```python
from build123d import *
from OCP.BRepFilletAPI import BRepFilletAPI_MakeChamfer

# Parameters (mm, degrees)
SKETCH9_R                    = 2
BOSS_EXTRUDE3_DEPTH          = 16
SKETCH10_R                   = 2
CUT_EXTRUDE7_DEPTH           = 14
SKETCH11_W                   = 7
SKETCH11_H                   = 26.686138344
CUT_EXTRUDE8_DEPTH           = 28
FILLET1_R                    = 2
CHAMFER1_SIZE                = 2.5
CHAMFER1_SIZE2               = 4.365846821
CHAMFER1_SIZE2_2             = 4.330127019
EXTRUDE1_DEPTH               = 3
EXTRUDE1_DEPTH_BACK          = 3
FILLET2_R                    = 2
FILLET3_R                    = 5
ESTRUSIONE_ESTRUSIONE1_DEPTH = 4.5
ESTRUSIONE_ESTRUSIONE2_DEPTH = 4.5


with BuildPart() as part:
    # Sketch9 → Boss-Extrude3 (new body)
    with BuildSketch(Plane(origin=(0, 0, 0), x_dir=(0, 0, -1), z_dir=(1, 0, 0))):
        with BuildLine():
            Line((8, 5.053889445), (8, -49.642014822))
            Line((8, -49.642014822), (-8, -49.642014822))
            Line((-8, -49.642014822), (-8, -10.875806049))
            ThreePointArc((-8, -10.875806049), (-8.427714838, -7.982476346), (-9.674271354, -5.336650652))
            ThreePointArc((-9.674271354, -5.336650652), (-7.418447874, 8.870328147), (6.925281884, 7.78202542))
            ThreePointArc((6.925281884, 7.78202542), (7.721634556, 6.519985019), (8, 5.053889445))
        make_face()
        Circle(SKETCH9_R, mode=Mode.SUBTRACT)
        with BuildLine():
            Line((5.5, -41.5), (5.5, -25.762364524))
            ThreePointArc((5.5, -25.762364524), (3.987567872, -22.111030369), (0.336233717, -20.598598241))
            Line((0.336233717, -20.598598241), (-0.410415455, -20.598598241))
            ThreePointArc((-0.410415455, -20.598598241), (-4.070351606, -22.119652678), (-5.574124284, -25.786723302))
            Line((-5.574124284, -25.786723302), (-5.5, -41.5))
            Line((-5.5, -41.5), (5.5, -41.5))
        make_face(mode=Mode.SUBTRACT)
    extrude(amount=BOSS_EXTRUDE3_DEPTH)

    # Sketch10 → Cut-Extrude7 (cut)
    with BuildSketch(Plane.XZ.offset(49.642014822)):
        with Locations(Location((8, 0, 0), (0, 0, 270))):
            Circle(SKETCH10_R)
    extrude(amount=-CUT_EXTRUDE7_DEPTH, mode=Mode.SUBTRACT)

    # Sketch11 → Cut-Extrude8 (cut)
    with BuildSketch(Plane(origin=(0, 16, 0), x_dir=(1, 0, 0), z_dir=(0, 1, 0))):
        with Locations((8, -2.737831409)):
            Rectangle(SKETCH11_W, SKETCH11_H)
    extrude(amount=-CUT_EXTRUDE8_DEPTH, mode=Mode.SUBTRACT)

    # Fillet1
    fillet1_edges = [part.edges().sort_by_distance(p)[0] for p in [
        (8, -49.642014822, 8),
        (8, -49.642014822, -8),
    ]]
    fillet(fillet1_edges, radius=FILLET1_R)

    # Chamfer1: one chamfer whose edges measure the first distance from different faces: ONE call of the kernel's chamfer builder (chamfer() names one face for all edges)
    chamfer1_edges_1 = [part.edges().sort_by_distance(p)[0] for p in [
        (8, -41.5, 5.5),
    ]]
    chamfer1_side_1 = [part.faces().sort_by_distance(p)[0] for p in [
        (8, -41.5, 5.305835122),
    ]]
    chamfer1_edges_2 = [part.edges().sort_by_distance(p)[0] for p in [
        (8, -41.5, -5.5),
    ]]
    chamfer1_side_2 = [part.faces().sort_by_distance(p)[0] for p in [
        (8, -41.5, 5.305835122),
    ]]
    chamfer1 = BRepFilletAPI_MakeChamfer(part.part.solid().wrapped)
    for e in chamfer1_edges_1:
        chamfer1.Add(CHAMFER1_SIZE, CHAMFER1_SIZE2, e.wrapped, chamfer1_side_1[0].wrapped)  # the first distance lies on this face
    for e in chamfer1_edges_2:
        chamfer1.Add(CHAMFER1_SIZE, CHAMFER1_SIZE2_2, e.wrapped, chamfer1_side_2[0].wrapped)  # the first distance lies on this face
    add(Compound.cast(chamfer1.Shape()), mode=Mode.REPLACE)

    # Sketch12 → Extrude1 (cut, two sides)
    with BuildSketch(Plane(origin=(0, -41.5, 0), x_dir=(1, 0, 0), z_dir=(0, 1, 0))) as extrude1_sk:
        Polygon((6.895214346, 4.750578313), (3.333485671, 1.418516714), (4.438271325, -3.332061599), (9.104785654, -4.750578313), (12.666514329, -1.418516714), (11.561728675, 3.332061599), align=None)
    extrude(amount=EXTRUDE1_DEPTH, mode=Mode.SUBTRACT)
    extrude(extrude1_sk.sketch, amount=-EXTRUDE1_DEPTH_BACK, mode=Mode.SUBTRACT)

    # Fillet2
    fillet2_edges = [part.edges().sort_by_distance(p)[0] for p in [
        (4.5, -12, 0),
        (11.5, -12, 0),
    ]]
    fillet(fillet2_edges, radius=FILLET2_R)

    # Fillet3
    fillet3_edges = [part.edges().sort_by_distance(p)[0] for p in [
        (8, -37.169872981, -5.5),
        (8, -37.134201755, 5.520594792),
    ]]
    fillet(fillet3_edges, radius=FILLET3_R)

    # Schizzo1 → Estrusione-Estrusione1 (add)
    with BuildSketch(Plane.ZY):
        Polygon((0.837135677, 11.156995776), (-8, 11.156995776), (-8, 4.232261394), (1.127037183, 4.232261394), align=None)
    extrude(amount=-ESTRUSIONE_ESTRUSIONE1_DEPTH)

    # Schizzo2 → Estrusione-Estrusione2 (add)
    with BuildSketch(Plane(origin=(16, 0, 0), x_dir=(0, 0, -1), z_dir=(1, 0, 0))):
        Polygon((-0.837135677, 11.156995776), (8, 11.156995776), (8, 3.955668155), (-3.77094248, 6.198951123), (-1.212549738, 11.150354711), align=None)
    extrude(amount=-ESTRUSIONE_ESTRUSIONE2_DEPTH)


solid = part.part
```
Could you check a few things on this model? Use its own coordinates, in mm. A direction names the side the tool comes from. Coordinates: 2 decimals unless noted, no trailing zeros. Loops run counter-clockwise (first coordinate to the right, second up) from the corner with the lowest first, then second, coordinate; pieces in that order, holes last. Notation, with made-up numbers: M -23.5,18.5 L 12.5,18.5 A20 cw 12.5,41.5 Z; hole C -38.75,63.25 d9. An arc over 180 degrees is marked long. Put each result on its own line as item: value. Start each with the question number.
(1) Suppose I cut it at D-D on x = 8. Please give me the cut outline in (y, z), then the cut area to 3 significant figures.
(2) Suppose I cut it at C-C on z = 7. Please give me the cut outline in (x, y), then the cut area to 3 significant figures.
(3) Will these pins go through, and if not, where does the flat tip stop? P1, Ø4.5, axis at y = 0, z = 0, coming from the -X side; P2, Ø3, axis at x = 5.5, y = -31, coming from the +Z side; P3, Ø0.8, axis at x = 7, z = 0, coming from the -Y side; P4, Ø4, axis at x = 13, y = 4, coming from the +Z side.
(4) Thinking about a two-plate mould opening in Z: for faces 4 (the face through (10, -47, 0)), 5 (the face through (13.616, -8.022, 8.416)), 6 (the face through (4.5, -2, 2)), which applies, pulls with the +Z half, pulls with the -Z half, needs draft (parallel to the pull), parting line crosses it, or undercut?
(5) Suppose I cut it at A-A on y = -22.5. Please give me the cut outline in (x, z), then the cut area to 3 significant figures.
(6) Suppose I cut it at B-B on y = 0. Please give me the cut outline in (x, z), then the cut area to 3 significant figures.
(7) For faces 1 (the face through (9.26, -42.21, -4.03)), 2 (the face through (10.9, -11.43, -0.09)), 3 (the face through (7.89, -38.8, 4.56)), which set-ups out of +Z, -Z, +X, -X, +Y, -Y let a thin tool reach every point of the face, with its end or its side?
(8) I need wall thicknesses on line 1 (Y direction, x = 15.05, z = 0); line 2 (X direction, y = 1, z = 6.5); line 3 (Z direction, x = 10.5, y = -35). Which ranges of each line are inside material? Lowest first, please. Write a range as from..to.
Solutions:
1. outline: M -49.64,-6 A2 ccw -47.64,-8 L -12,-8 L -12,8 L -47.64,8 A2 ccw -49.64,6 L -49.64,2 L -44.5,2 L -44.5,4.41 L -39.05,4.41 L -38.28,4.86 A5 cw -35.81,5.53 L -25.79,5.57 A5.16 cw -20.6,0.41 L -20.6,-0.34 A5.16 cw -25.76,-5.5 L -35.83,-5.5 A5 cw -38.33,-4.83 L -39.05,-4.41 L -44.5,-4.41 L -44.5,-2 L -49.64,-2 Z
1. area: 342 mm2
2. outline: M 0,-49.37 L 16,-49.37 L 16,9.18 L 11.5,9.18 L 11.5,-10 A2 cw 9.5,-12 L 6.5,-12 A2 cw 4.5,-10 L 4.5,9.18 L 0,9.18 Z
2. area: 790 mm2
3. P1: stops at x = 0
3. P2: stops at z = 8
3. P3: stops at y = -20.6
3. P4: stops at z = 11.35
4. face 4: undercut
4. face 5: pulls with the +Z half
4. face 6: needs draft
5. outline: M 0,-8 L 16,-8 L 16,-4.34 L 0,-4.34 Z; M 0,4.41 L 16,4.41 L 16,8 L 0,8 Z
5. area: 116 mm2
6. outline: M 0,-8 L 4.5,-8 L 4.5,-2 L 0,-2 Z; M 0,2 L 4.5,2 L 4.5,11.44 L 0,11.44 Z; M 11.5,-8 L 16,-8 L 16,-2 L 11.5,-2 Z; M 11.5,2 L 16,2 L 16,11.44 L 11.5,11.44 Z
6. area: 139 mm2
7. face 1: none
7. face 2: +Z, -Z, +Y
7. face 3: +X, -X
8. line 1: y = -49.64..-41.5, -20.6..-2, 2..11.16
8. line 2: x = 0..4.5, 11.5..16
8. line 3: z = -8..-5.5, 5.53..8
